Could you check a few things on this model? Use its own coordinates, in mm. Coordinates: 2 decimals unless noted, no trailing zeros. Loops run counter-clockwise (first coordinate to the right, second up) from the corner with the lowest first, then second, coordinate; pieces in that order, holes last.
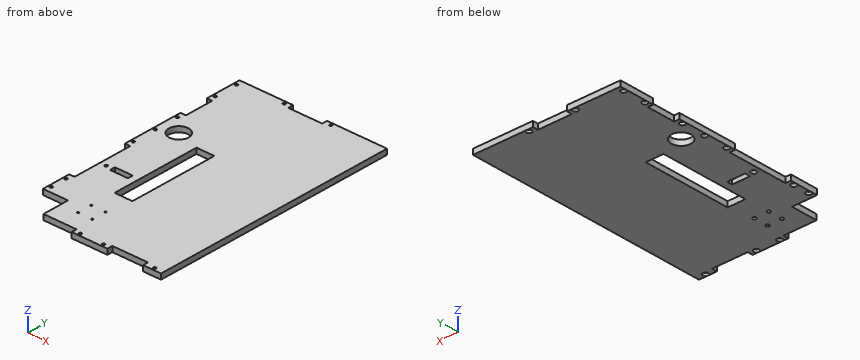
from build123d import *

# Parameters (mm, degrees)
ESQUISSE1_W             = 165
ESQUISSE1_H             = 276
BOSS_EXTRU_1_DEPTH      = 6
ESQUISSE2_W             = 38
ESQUISSE2_H             = 6
ESQUISSE2_W_2           = 6
ESQUISSE2_H_2           = 32
ESQUISSE2_H_3           = 68
ESQUISSE2_W_3           = 40
EXTERIEUR_DEPTH         = 10
ESQUISSE3_R             = 11
ESQUISSE3_W             = 20
ESQUISSE3_H             = 6
ENL_V_MAT_EXTRU_2_DEPTH = 322.616230934
ESQUISSE4_R             = 1.5
ESQUISSE4_R_2           = 1.005
ENL_V_MAT_EXTRU_3_DEPTH = 322.616230934
ESQUISSE5_R             = 2.995
ESQUISSE5_R_2           = 3
ESQUISSE5_R_3           = 2
ENL_V_MAT_EXTRU_4_DEPTH = 3
ESQUISSE6_W             = 20
ESQUISSE6_H             = 100
ENL_V_MAT_EXTRU_5_DEPTH = 322.616230934


with BuildPart() as part:
    # Esquisse1 → Boss.-Extru.1 (new body)
    with BuildSketch(Plane.XY):
        with Locations((-82.5, 138)):
            Rectangle(ESQUISSE1_W, ESQUISSE1_H)
    extrude(amount=BOSS_EXTRU_1_DEPTH)

    # Esquisse2 → exterieur (cut)
    with BuildSketch(Plane.XY.offset(6)):
        with Locations((-86, 273)):
            Rectangle(ESQUISSE2_W, ESQUISSE2_H)
        with Locations((-162, 220)):
            Rectangle(ESQUISSE2_W_2, ESQUISSE2_H_2)
        with Locations((-162, 102)):
            Rectangle(ESQUISSE2_W_2, ESQUISSE2_H_3)
        Polygon((-137, 36), (-137, 6), (-100, 6), (-100, 0), (-165, 0), (-165, 36), align=None)
        with Locations((-40, 3)):
            Rectangle(ESQUISSE2_W_3, ESQUISSE2_H)
    extrude(amount=-EXTERIEUR_DEPTH, mode=Mode.SUBTRACT)

    # Esquisse3 → Enlèv. mat.-Extru.2 (cut, through all)
    with BuildSketch(Plane.XY.offset(6)):
        with Locations((-144, 178.92)):
            Circle(ESQUISSE3_R)
        with Locations((-135, 99)):
            Rectangle(ESQUISSE3_W, ESQUISSE3_H)
    extrude(amount=-ENL_V_MAT_EXTRU_2_DEPTH, mode=Mode.SUBTRACT)

    # Esquisse4 → Enlèv. mat.-Extru.3 (cut, through all)
    with BuildSketch(Plane.XY.offset(6)):
        with Locations((-60, 273)):
            Circle(ESQUISSE4_R)
        with Locations((-112, 273)):
            Circle(ESQUISSE4_R)
        with Locations((-162, 197)):
            Circle(ESQUISSE4_R)
        with Locations((-162, 170)):
            Circle(ESQUISSE4_R)
        with Locations((-162, 143)):
            Circle(ESQUISSE4_R)
        with Locations((-162, 61)):
            Circle(ESQUISSE4_R)
        with Locations((-162, 43)):
            Circle(ESQUISSE4_R)
        with Locations((-93, 3)):
            Circle(ESQUISSE4_R)
        with Locations((-67, 3)):
            Circle(ESQUISSE4_R)
        with Locations((-10, 3)):
            Circle(ESQUISSE4_R)
        with Locations((-162, 269)):
            Circle(ESQUISSE4_R)
        with Locations((-162, 243)):
            Circle(ESQUISSE4_R)
        with Locations((-117.5, 27)):
            Circle(ESQUISSE4_R_2)
        with Locations((-117.5, 43)):
            Circle(ESQUISSE4_R_2)
        with Locations((-101.5, 43)):
            Circle(ESQUISSE4_R_2)
        with Locations((-101.5, 27)):
            Circle(ESQUISSE4_R_2)
        with Locations((-152, 99)):
            Circle(ESQUISSE4_R)
    extrude(amount=-ENL_V_MAT_EXTRU_3_DEPTH, mode=Mode.SUBTRACT)

    # Esquisse5 → Enlèv. mat.-Extru.4 (cut)
    with BuildSketch(Plane(origin=(0, 0, 0), x_dir=(-1, 0, 0), z_dir=(0, 0, -1))):
        with Locations((60, 273)):
            Circle(ESQUISSE5_R)
        with Locations((112, 273)):
            Circle(ESQUISSE5_R)
        with Locations((162, 197)):
            Circle(ESQUISSE5_R)
        with Locations((162, 170)):
            Circle(ESQUISSE5_R)
        with Locations((162, 143)):
            Circle(ESQUISSE5_R)
        with Locations((162, 61)):
            Circle(ESQUISSE5_R)
        with Locations((162, 43)):
            Circle(ESQUISSE5_R)
        with Locations((93, 3)):
            Circle(ESQUISSE5_R)
        with Locations((67, 3)):
            Circle(ESQUISSE5_R)
        with Locations((10, 3)):
            Circle(ESQUISSE5_R)
        with Locations((162, 269)):
            Circle(ESQUISSE5_R)
        with Locations((162, 243)):
            Circle(ESQUISSE5_R)
        with Locations((152, 99)):
            Circle(ESQUISSE5_R_2)
        with Locations((117.5, 43)):
            Circle(ESQUISSE5_R_3)
        with Locations((117.5, 27)):
            Circle(ESQUISSE5_R_3)
        with Locations((101.5, 27)):
            Circle(ESQUISSE5_R_3)
        with Locations((101.5, 43)):
            Circle(ESQUISSE5_R_3)
    extrude(amount=-ENL_V_MAT_EXTRU_4_DEPTH, mode=Mode.SUBTRACT)

    # Esquisse6 → Enlèv. mat.-Extru.5 (cut, through all)
    with BuildSketch(Plane(origin=(0, 0, 0), x_dir=(-1, 0, 0), z_dir=(0, 0, -1))):
        with Locations((107, 121)):
            Rectangle(ESQUISSE6_W, ESQUISSE6_H)
    extrude(amount=-ENL_V_MAT_EXTRU_5_DEPTH, mode=Mode.SUBTRACT)


solid = part.part
(1) I need wall thicknesses on probe 1 along Y at (x, z) = (-144, 2.85); probe 2 along Y at (x, z) = (-98, 5.25); probe 3 along X at (y, z) = (273, 1.95) (3 decimals). Which ranges of each line are inside material? Lowest first, please.
Answers:
probe 1: y = 36 to 96, 102 to 167.92, 189.92 to 276
probe 2: y = 0 to 71, 171 to 270
probe 3: x = -165 to -114.995, -109.005 to -105, -67 to -62.995, -57.005 to 0
(2) Imagine slicing it at A-A, the plane y = 158.5. Write out the boundary of the cut face in (x, z).
Answers:
outline: (-165, 0) - (-117, 0) - (-117, 6) - (-165, 6) - close; (-97, 0) - (0, 0) - (0, 6) - (-97, 6) - close
(3) Imagine slicing it at C-C, the plane z = 4.4. State how many separate pieces and enclosed holes the cut face has, and give its area (3 significant figures).
Answers:
separate pieces: 1
enclosed holes: 20
area: 40,600 mm2
(4) Imagine slicing it at B-B, the plane x = -74. Write out the boundary of the cut face in (y, z).
Answers:
outline: (0, 0) - (270, 0) - (270, 6) - (0, 6) - close
(5) For pin 1 (5.5 mm diameter, centred on x = -162, y = 269, fed in from -Z); pin 2 (6.5 mm diameter, centred on x = -150.5, y = 99.5, fed in from -Z); pin 3 (3 mm diameter, centred on x = -89.5, z = 1, fed in from +Y), each with a flat end and sliding along its axis, tell me the tip position at first contact or that it passes through.
Answers:
pin 1: stops at z = 3
pin 2: stops at z = 0
pin 3: stops at y = 270
